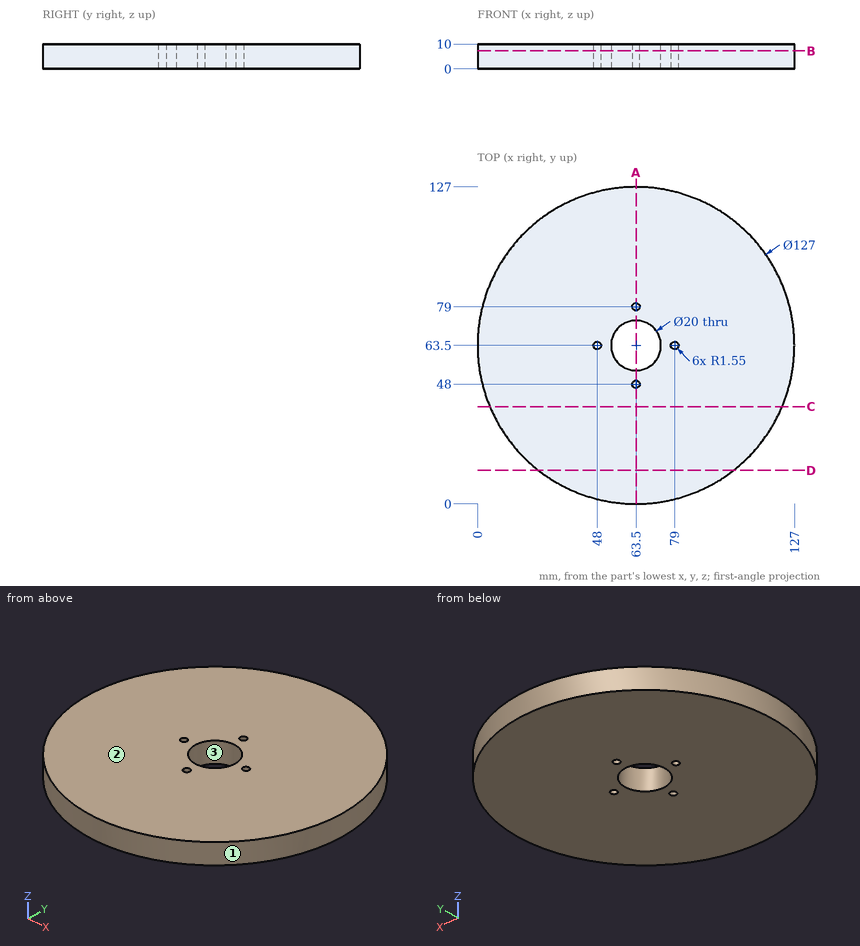
The figure shows three views and two pictorial views of one solid part (mm, origin at its lowest corner). Answer the questions. Give positions to 0.01 mm unless a question says otherwise; leave off trailing zeros. Write each loop counter-clockwise with the first axis right and the second up, starting at its lowest first coordinate (ties: lowest second). Pieces come first, ordered by that corner, then holes. Notation, with made-up numbers: (60.25, -10.75) -> (69.25, -10.75) arc R23 cw to (69.25, 18.25) -> close; hole circle Ø8 at (-21.5, 3). An arc over 180 degrees is marked (long way). Use one line per item in the form item = value.
1) For a pull along X with two mould halves and no side action, classify the marked faces 1, 2 and 3 as +X half, -X half, draft (parallel to the pull), parting line (faces both ways), or undercut.
Result:
face_1 = parting line
face_2 = draft
face_3 = undercut
2) Straight lines are drawn through the part: probe 1 along Y at (x, z) = (63.5, 4.5); probe 2 along Y at (x, z) = (57.5, 6.5) (1 decimal); probe 3 along Y at (x, z) = (86, 3.75). For each, find the intervals that lie inside material, in ascending order.
Result:
probe_1 = 0 to 46.45, 49.55 to 53.5, 73.5 to 77.45, 80.55 to 127
probe_2 = 0.3 to 55.5, 71.5 to 126.7
probe_3 = 4.12 to 122.88
3) Section A-A on x = 63.5 is taken. Write down the section's boundary in (y, z), plus the area to 3 significant figures.
Result:
outline = (0, 0) -> (46.45, 0) -> (46.45, 10) -> (0, 10) -> close; (49.55, 0) -> (53.5, 0) -> (53.5, 10) -> (49.55, 10) -> close; (73.5, 0) -> (77.45, 0) -> (77.45, 10) -> (73.5, 10) -> close; (80.55, 0) -> (127, 0) -> (127, 10) -> (80.55, 10) -> close
area = 1,010 mm²
4) Section D-D on y = 13.5 is taken. Write down the section's boundary in (x, z), plus the area to 3 significant figures.
Result:
outline = (24.36, 0) -> (102.64, 0) -> (102.64, 10) -> (24.36, 10) -> close
area = 783 mm²
5) Section C-C on y = 39 is taken. Write down the section's boundary in (x, z).
Result:
outline = (4.92, 0) -> (122.08, 0) -> (122.08, 10) -> (4.92, 10) -> close
6) Each of these flat-tipped pins is pushed along its axis until it touches: P1, Ø1, axis at x = 110.5, y = 38, coming from the -Z side; P2, Ø1, axis at y = 68, z = 4.5, coming from the +X side; P3, Ø1.5, axis at x = 56, y = 59, coming from the -Z side; P4, Ø5, axis at x = 86, z = 1.5, coming from the -Y side. Where does it stop, or does it pass through?
Result:
P1 = 0
P2 = 126.87
P3 = through
P4 = 3.23
7) Section B-B on z = 7.25 is taken. Write down the section's boundary in (x, y), plus the area to 3 significant figures.
Result:
outline = circle Ø127 at (63.5, 63.5); hole (48.08, 61.95) arc R1.55 ccw to (49.55, 63.5) arc R1.55 ccw to (48.08, 65.05) arc R1.55 ccw (long way) to start; hole circle Ø20 at (63.5, 63.5); hole (65.05, 48) arc R1.55 ccw to (65.05, 48.08) arc R1.55 ccw (long way) to start; hole (65.05, 78.92) arc R1.55 ccw to (65.05, 79) arc R1.55 ccw (long way) to start; hole (78.92, 61.95) arc R1.55 ccw to (80.55, 63.5) arc R1.55 ccw to (78.92, 65.05) arc R1.55 ccw to start
area = 12,300 mm²
